from build123d import *

# Parameters (mm, degrees)
SKETCH1_R              = 3.7592
BOSS_EXTRUDE1_DEPTH    = 1.5875
FILLET1_R              = 5.08
FILLET2_R              = 1.27
SKETCH3_W              = 1.5875
SKETCH3_H              = 9.2075
CUT_EXTRUDE1_DEPTH     = 23.437165875
WEIGHT_REDUCTION_REACH = 24.437
FILLET3_R              = 2.54


with BuildPart() as part:
    # Sketch1 → Boss-Extrude1 (new body)
    with BuildSketch(Plane.XY):
        with BuildLine():
            Line((11.1125, 17.8308), (9.525, 17.8308))
            Line((9.525, 17.8308), (9.525, 19.05))
            Line((9.525, 19.05), (2.54, 19.05))
            ThreePointArc((2.54, 19.05), (-6.440256121, 15.330256121), (-10.16, 6.35))
            Line((-10.16, 6.35), (-10.16, 2.5908))
            Line((-10.16, 2.5908), (-11.7475, 2.5908))
            Line((-11.7475, 2.5908), (-11.7475, 1.27))
            Line((-11.7475, 1.27), (-10.16, 1.27))
            Line((-10.16, 1.27), (-10.16, -14.605))
            Line((-10.16, -14.605), (9.525, -14.605))
            Line((9.525, -14.605), (9.525, -6.4008))
            Line((9.525, -6.4008), (11.1125, -6.4008))
            Line((11.1125, -6.4008), (11.1125, -5.08))
            Line((11.1125, -5.08), (9.525, -5.08))
            Line((9.525, -5.08), (9.525, 2.54))
            Line((9.525, 2.54), (11.1125, 2.54))
            Line((11.1125, 2.54), (11.1125, 3.8608))
            Line((11.1125, 3.8608), (9.525, 3.8608))
            Line((9.525, 3.8608), (9.525, 16.51))
            Line((9.525, 16.51), (11.1125, 16.51))
            Line((11.1125, 16.51), (11.1125, 17.8308))
        make_face()
        Circle(SKETCH1_R, mode=Mode.SUBTRACT)
    extrude(amount=BOSS_EXTRUDE1_DEPTH)

    # Fillet1
    fillet1_edges = [part.edges().sort_by_distance(p)[0] for p in [
        (9.525, -14.605, 0.79375),
    ]]
    fillet(fillet1_edges, radius=FILLET1_R)

    # Fillet2
    fillet2_edges = [part.edges().sort_by_distance(p)[0] for p in [
        (-10.16, -14.605, 0.79375),
    ]]
    fillet(fillet2_edges, radius=FILLET2_R)

    # Sketch3 → Cut-Extrude1 (cut, through all)
    with BuildSketch(Plane(origin=(0, 0, 0), x_dir=(-1, 0, 0), z_dir=(0, 0, -1))):
        with Locations((6.19125, 14.44625)):
            Rectangle(SKETCH3_W, SKETCH3_H)
    extrude(amount=-CUT_EXTRUDE1_DEPTH, mode=Mode.SUBTRACT)

    # Sketch2 → Weight Reduction (cut, up to next)
    with BuildSketch(Plane.XY.offset(1.5875), mode=Mode.PRIVATE) as weight_reduction_sk1:
        with BuildLine():
            Line((-3.4925, 13.884590085), (5.715, 2.384426271))
            Line((5.715, 2.384426271), (5.715, 16.002))
            Line((5.715, 16.002), (2.54, 16.002))
            ThreePointArc((2.54, 16.002), (-0.656657668, 15.457276418), (-3.4925, 13.884590085))
        make_face()
    weight_reduction_tool1 = extrude(weight_reduction_sk1.sketch, amount=-WEIGHT_REDUCTION_REACH, mode=Mode.PRIVATE) & part.part
    add(weight_reduction_tool1.solids().sort_by_distance((2.48474, 11.130093, 1.5875))[0], mode=Mode.SUBTRACT)

    # Fillet3
    fillet3_edges = [part.edges().sort_by_distance(p)[0] for p in [
        (5.715, 16.002, 0.79375),
        (5.715, 2.384426271, 0.79375),
        (-3.4925, 13.884590085, 0.79375),
    ]]
    fillet(fillet3_edges, radius=FILLET3_R)


solid = part.part
Here's how the part is built. I have some questions about the finished solid (model axes, mm). A direction names the side the tool comes from. Coordinates: 2 decimals unless noted, no trailing zeros. Order: outer loops, then holes, each group sorted by start corner. A loop starts at its lowest first (then second) coordinate and runs counter-clockwise, first axis right, second up. Notation, with made-up numbers: (-12, -4) -> (24, -4) arc R15 cw to (24, 4) -> close; hole circle Ø8 at (14.25, 45). An arc over 180 degrees is marked (long way). Answer in a Markdown table with one row per item.
(1) I want a section at C-C on z = 1.2. Count the separate pieces of the cut face and the enclosed holes in it, then the cut area to 3 significant figures.
Answer key:
| item | result |
|---|---|
| separate pieces | 1 |
| enclosed holes | 2 |
| area | 523 mm^2 |
(2) Will these pins go through, and if not, where does the flat tip stop? pin 1 Ø0.8 at (x, z) = (10, 1) entering from -Y; pin 2 Ø0.5 at (y, z) = (-0.5, 1) entering from +X (3 decimals); pin 3 Ø0.5 at (x, z) = (-11, 1) entering from -Y.
Answer key:
| item | result |
|---|---|
| pin 1 | y = -6.4 |
| pin 2 | x = 9.525 |
| pin 3 | y = 1.27 |
(3) Please list where these lines run through material, in increasing order: probe 1 along Y at (x, z) = (9.75, 0.55); probe 2 along Y at (x, z) = (-1.25, 0.75) (3 decimals); probe 3 along X at (y, z) = (13, 1.5) (1 decimal).
Answer key:
| item | result |
|---|---|
| probe 1 | -6.4 to -5.08, 2.54 to 3.86, 16.51 to 17.83 |
| probe 2 | -14.605 to -3.545, 3.545 to 11.084, 15.079 to 18.471 |
| probe 3 | -8.3 to -7, -5.4 to -2.2, 5.7 to 9.5 |
(4) I want a section at D-D on y = -4.5. List the corners of the cut face in (x, z) for me (1 decimal).
Answer key:
| item | result |
|---|---|
| outline | (-10.2, 0) -> (9.5, 0) -> (9.5, 1.6) -> (-10.2, 1.6) -> close |
(5) I want a section at A-A on x = 0. List the corners of the cut face in (y, z) for me (1 decimal), then the cut area to 3 significant figures.
Answer key:
| item | result |
|---|---|
| outline | (-14.6, 0) -> (-3.8, 0) -> (-3.8, 1.6) -> (-14.6, 1.6) -> close; (3.8, 0) -> (9.5, 0) -> (9.5, 1.6) -> (3.8, 1.6) -> close; (15.7, 0) -> (18.8, 0) -> (18.8, 1.6) -> (15.7, 1.6) -> close |
| area | 31.3 mm^2 |
(6) On a 3-axis mill with a long thin cutter (end or side, diameter ignored), from which of +Z, -Z, +X, -X, +Y, -Y can I reach the whole of each face in a straight line? I mean faces 1 (the face through (9.525, -1, 1)), 2 (the face through (-6, 9.842, 1)), 3 (the face through (9.525, 18, 1)), 4 (the face through (5.715, 12, 1)). Say none if no direction works.
Answer key:
| item | result |
|---|---|
| face 1 | +Z, -Z, +X |
| face 2 | +Z, -Z, +Y |
| face 3 | +Z, -Z, +X, +Y |
| face 4 | +Z, -Z |
(7) Thinking about a two-plate mould opening in X: for faces 5 (the face through (10, 16.51, 1)), 6 (the face through (9.525, 10, 1)), 7 (the face through (-5.398, 13, 1)), 8 (the face through (-2.05, 13.89, 0.78)), which applies, +X half, -X half, draft (parallel to the pull), parting line (faces both ways), or undercut?
Answer key:
| item | result |
|---|---|
| face 5 | draft |
| face 6 | +X half |
| face 7 | undercut |
| face 8 | undercut |
(8) I want a section at B-B on y = -1. List the corners of the cut face in (x, z) for me (1 decimal), then the cut area to 3 significant figures.
Answer key:
| item | result |
|---|---|
| outline | (-10.2, 0) -> (-3.6, 0) -> (-3.6, 1.6) -> (-10.2, 1.6) -> close; (3.6, 0) -> (9.5, 0) -> (9.5, 1.6) -> (3.6, 1.6) -> close |
| area | 19.7 mm^2 |
